from build123d import *

# Parameters (mm, degrees)
F1_DEPTH = 114.3
F2_R     = 5.08
F3_R     = 17.78


with BuildPart() as f1:
    # F0 (on Front) → F1 (new body)
    with BuildSketch(Plane.XZ):
        with BuildLine():
            ThreePointArc((218.44, 133.495064), (0, 185.76179), (-218.44, 133.495064))
            Line((-218.44, 133.495064), (-205.74, 113.457282))
            ThreePointArc((-205.74, 113.457282), (0, 162.364627), (205.74, 113.457282))
            Line((205.74, 113.457282), (218.44, 133.495064))
        make_face()
    extrude(amount=-F1_DEPTH)

    # F2
    f2_edges = [f1.edges().sort_by_distance(p)[0] for p in [
        (0, 0, 185.76179),
        (0, 114.3, 162.364627),
        (0, 114.3, 185.76179),
    ]]
    fillet(f2_edges, radius=F2_R)

    # F3
    f3_edges = [f1.edges().sort_by_distance(p)[0] for p in [
        (0, 0, 162.364627),
    ]]
    fillet(f3_edges, radius=F3_R)


solid = f1.part
Could you check a few things on this model? Use its own coordinates, in mm. Coordinates: 2 decimals unless noted, no trailing zeros. Write each loop counter-clockwise with the first axis right and the second up, starting at its lowest first coordinate (ties: lowest second). Pieces come first, ordered by that corner, then holes. Notation, with made-up numbers: (14, -20.5) - (22, -20.5) arc R22 cw to (22, 14.5) - close; hole circle Ø1 at (63, 81). An arc over 180 degrees is marked (long way). Put each result on its own line as item: value. Start each with the question number.
Q1. Please list where these lines run through material, in increasing order: L1, parallel to X at y = 97, z = 120; L2, parallel to X at y = 103, z = 130.5; L3, parallel to Z at x = -70, y = 14.
Q2. Thinking about a two-plate mould opening in X: for faces 1 (the cylindrical face through (-2.988, 62.86, 162.355)), 2 (the flat face through (212.001, 56.35, 123.336)), 3 (the cylindrical face through (3.17, 56.42, 185.75)), which applies, pulls with the +X half, pulls with the -X half, needs draft (parallel to the pull), parting line crosses it, or undercut?
Q3. I'm going to push flat-ended pins straight in: P1, Ø1, axis at x = -89.5, y = 38.5, coming from the -Z side; P2, Ø2, axis at x = -157.5, y = 23.5, coming from the +Z side; P3, Ø12, axis at x = 85, z = 153.5, coming from the -Y side. Where does each tip first touch, or does it pass through?
Q4. I want a section at A-A on y = 33.5. Write out the boundary of the cut face in (x, z), plus the area to 3 significant figures.
Checks:
1. L1: -209.89 to -192.21, 192.21 to 209.89
1. L2: -216.54 to -167.7, 167.7 to 216.54
1. L3: 157.39 to 180.66
2. face 1: undercut
2. face 2: pulls with the +X half
2. face 3: parting line crosses it
3. P1: z = 153.42
3. P2: z = 159.68
3. P3: y = 5.29
4. outline: (-218.44, 133.5) - (-205.74, 113.46) arc R457.2 cw to (205.74, 113.46) - (218.44, 133.5) arc R482.6 ccw to start
4. area: 10,300 mm²
